Input: part model. Units: mm. Frame: model coordinates. Face numbers are marked on the shaded views. A direction names the side the tool comes from. Round coordinates to 2 decimals unless told otherwise and drop trailing zeros. Write each loop counter-clockwise with the first axis right and the second up, starting at its lowest first coordinate (ties: lowest second). Pieces come first, ordered by that corner, then holes. Notation, with made-up numbers: (0, 73) - (10, 73) arc R23 cw to (10, 100) - close; hole circle Ø11 at (-2, -12). An arc over 180 degrees is marked (long way). One line per item, written item: value. Start each with the question number.
Solid Edge part; units mm, degrees
sketch "Sketch1" plane through (0, 0, 0) normal (0, -1, 0) x (1, 0, 0)
  line L0 (1469.4867, 25) -> (1469.4867, 0)
  line L1 (1469.4867, 0) -> (649.4867, 0)
  line L2 (649.4867, 0) -> (649.4867, 25)
  line L3 (649.4867, 25) -> (729.4867, 25)
  line L4 (729.4867, 25) -> (729.4867, 26.5)
  line L5 (729.4867, 26.5) -> (889.4867, 26.5)
  line L6 (889.4867, 26.5) -> (889.4867, 27.5)
  line L7 (889.4867, 27.5) -> (1029.4867, 27.5)
  line L8 (1029.4867, 27.5) -> (1029.4867, 28.5)
  line L9 (1029.4867, 28.5) -> (1099.4867, 28.5)
  line L10 (1099.4867, 28.5) -> (1099.4867, 30)
  line L11 (1099.4867, 30) -> (1179.4867, 30)
  line L12 (1179.4867, 30) -> (1179.4867, 28)
  line L13 (1179.4867, 28) -> (1249.4867, 28)
  line L14 (1249.4867, 28) -> (1249.4867, 26.5)
  line L15 (1249.4867, 26.5) -> (1389.4867, 26.5)
  line L16 (1389.4867, 26.5) -> (1389.4867, 25)
  line L17 (1389.4867, 25) -> (1469.4867, 25)
revolve "RevolvedProtrusion1" add sketch "Sketch1" angle 360 about axis through (0, 0, 0) along (1, 0, 0)
sketch "Sketch2" plane through (689.4867, -25, 0) normal (0, -1, 0) x (-1, 0, 0)
  line L0 (20, -8) -> (-35, -8)
  line L1 (-35, -8) -> (-35, 0)
  line L2 (-35, 0) -> (-35, 8)
  line L3 (-35, 8) -> (20, 8)
  line L4 (20, 8) -> (20, -8)
extrude "Cutout1" cut sketch "Sketch2" against normal blind 5
sketch "Sketch3" plane through (809.4867, -26.5, 0) normal (0, -1, 0) x (-1, 0, 0)
  line L0 (-75, 0) -> (-75, 8)
  line L1 (-75, 8) -> (-20, 8)
  line L2 (-20, 8) -> (-20, -8)
  line L3 (-20, -8) -> (-75, -8)
  line L4 (-75, -8) -> (-75, 0)
  dimension "D1" = 75
extrude "Cutout2" cut sketch "Sketch3" against normal blind 5
sketch "Sketch4" plane through (959.4867, -27.5, 0) normal (0, -1, 0) x (-1, 0, 0)
  line L0 (-65, 0) -> (-65, 8)
  line L1 (-65, 8) -> (-10, 8)
  line L2 (-10, 8) -> (-10, -8)
  line L3 (-10, -8) -> (-65, -8)
  line L4 (-65, -8) -> (-65, 0)
  dimension "D1" = 65
  dimension "D2" = 10
extrude "Keyway_Thickness" cut sketch "Sketch4" against normal blind 5
sketch "Sketch5" plane through (1064.4867, -28.5, 0) normal (0, -1, 0) x (-1, 0, 0)
  line L0 (-30, 0) -> (-30, 8)
  line L1 (-30, 8) -> (25, 8)
  line L2 (25, 8) -> (25, -8)
  line L3 (25, -8) -> (-30, -8)
  line L4 (-30, -8) -> (-30, 0)
  dimension "D1" = 30
  dimension "D2" = 25
extrude "Cutout3" cut sketch "Sketch5" against normal blind 5
sketch "Sketch6" plane through (1214.4867, -28, 0) normal (0, -1, 0) x (-1, 0, 0)
  line L0 (-25, 0) -> (-25, 8)
  line L1 (-25, 8) -> (30, 8)
  line L2 (30, 8) -> (30, -8)
  line L3 (30, -8) -> (-25, -8)
  line L4 (-25, -8) -> (-25, 0)
  dimension "D1" = 30
  dimension "D2" = 25
extrude "Cutout4" cut sketch "Sketch6" against normal blind 5
sketch "Sketch7" plane through (1319.4867, -26.5, 0) normal (0, -1, 0) x (-1, 0, 0)
  line L0 (65, 0) -> (65, 8)
  line L1 (65, 8) -> (10, 8)
  line L2 (10, 8) -> (10, -8)
  line L3 (10, -8) -> (65, -8)
  line L4 (65, -8) -> (65, 0)
  dimension "D1" = 65
  dimension "D2" = 10
extrude "Cutout5" cut sketch "Sketch7" against normal blind 5
sketch "Sketch8" plane through (1429.4867, -25, 0) normal (0, -1, 0) x (-1, 0, 0)
  line L0 (35, 0) -> (35, 8)
  line L1 (35, 8) -> (-20, 8)
  line L2 (-20, 8) -> (-20, -8)
  line L3 (-20, -8) -> (35, -8)
  line L4 (35, -8) -> (35, 0)
  dimension "D1" = 35
  dimension "D2" = 20
extrude "Cutout6" cut sketch "Sketch8" against normal blind 5
sketch "Sketch9" plane through (649.4867, 0, 0) normal (-1, 0, 0) x (0, -1, 0)
  circle A0 centre (0, 0) radius 25
extrude "Protrusion1" add sketch "Sketch9" along normal blind 25
sketch "Sketch10" plane through (1469.4867, 0, 0) normal (1, 0, 0) x (0, 0, 1)
  circle A0 centre (0, 0) radius 25
extrude "Protrusion2" add sketch "Sketch10" along normal blind 25
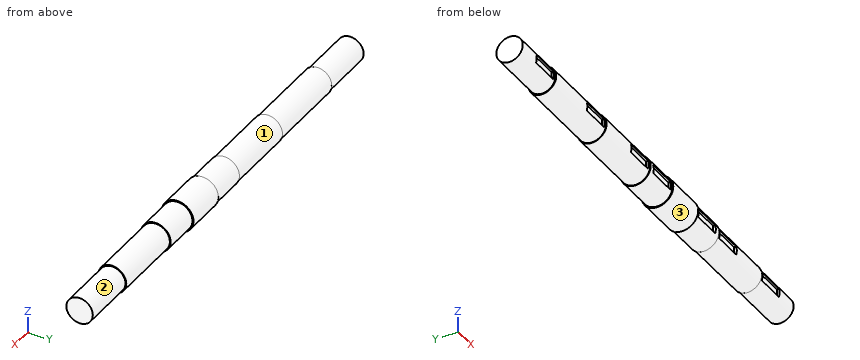
Q1. Access query for the marked faces 1, 2 and 3. Directions: +Z, -Z, +X, -X, +Y, -Y. A direction counts if a zero-diameter tool reaches every point of the face in a straight line with its end or side. Return the directions, or none.
Q2. Contact query for flat-ended pins moving along their axis: pin 1 Ø17.5 at (x, z) = (1061, 0.5) entering from -Y; pin 2 Ø1.1 at (x, y) = (853.5, -23) entering from +Z; pin 3 Ø3 at (x, y) = (1415, -22) entering from -Z. Output: stop coordinate, or through.
Q3. Cut plane D-D, the plane x = 858. Output: boundary loops of the cut face in (y, z).
Q4. Material intervals for probe 1 along X at (y, z) = (20, -21); probe 2 along Y at (x, z) = (951, 3); probe 3 along Z at (x, y) = (1223, -12.5), sorted ascending. Write a range as from..to.
Q5. Cut plane C-C, the plane x = 1107.5. Output: boundary loops of the cut face in (y, z).
Q6. Cut plane B-B, the plane x = 994.5. Output: boundary loops of the cut face in (y, z).
A:
1. face 1: -X
1. face 2: +X
1. face 3: +X, -X
2. pin 1: stops at y = -27.35
2. pin 2: stops at z = 14.08
2. pin 3: stops at z = -14.31
3. outline: (-25.26, -8) arc R26.5 ccw (long way) to (-25.26, 8) - (-21.5, 8) - (-21.5, -8) - close
4. probe 1: x = 1099.49..1179.49
4. probe 2: y = -27.34..27.34
4. probe 3: z = -25.05..25.05
5. outline: circle Ø60 at (0, 0)
6. outline: (-26.31, -8) arc R27.5 ccw (long way) to (-26.31, 8) - (-22.5, 8) - (-22.5, -8) - close
